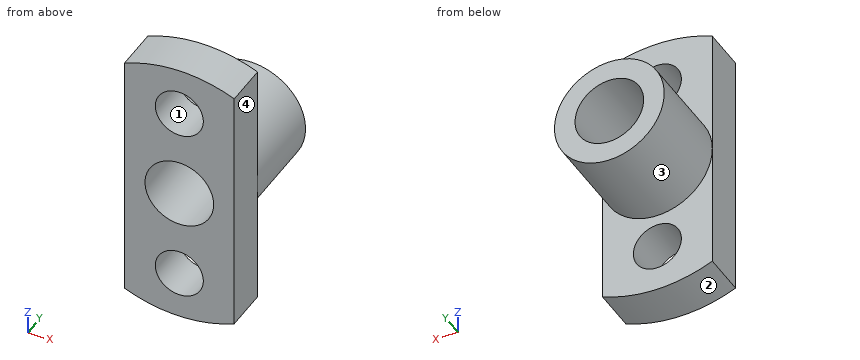
```python
from build123d import *

# Parameters (mm, degrees)
SKETCH_2_R          = 1.75
EXTRUDE_1_DEPTH     = 3.2
SKETCH_3_R          = 4
EXTRUDE_2_DEPTH     = 6.6
SKETCH_4_R          = 2.5
CUT_EXTRUDE_1_DEPTH = 10.8


with BuildPart() as part:
    # 草图2 → 凸台-拉伸1 (new body)
    with BuildSketch(Plane(origin=(0, 0, 0), x_dir=(1, 0, 0), z_dir=(0, 1, 0))):
        with BuildLine():
            Line((-4, 9.16515139), (-4, -9.16515139))
            ThreePointArc((-4, -9.16515139), (0, -10), (4, -9.16515139))
            Line((4, -9.16515139), (4, 9.16515139))
            ThreePointArc((4, 9.16515139), (0, 10), (-4, 9.16515139))
        make_face()
        with Locations((0, 6.5)):
            Circle(SKETCH_2_R, mode=Mode.SUBTRACT)
        with Locations((0, -6.5)):
            Circle(SKETCH_2_R, mode=Mode.SUBTRACT)
    extrude(amount=EXTRUDE_1_DEPTH)

    # 草图3 → 凸台-拉伸2 (add)
    with BuildSketch(Plane(origin=(0, 3.2, 0), x_dir=(1, 0, 0), z_dir=(0, 1, 0))):
        Circle(SKETCH_3_R)
    extrude(amount=EXTRUDE_2_DEPTH)

    # 草图4 → 切除-拉伸1 (cut, through all)
    with BuildSketch(Plane(origin=(0, 9.8, 0), x_dir=(1, 0, 0), z_dir=(0, 1, 0))):
        Circle(SKETCH_4_R)
    extrude(amount=-CUT_EXTRUDE_1_DEPTH, mode=Mode.SUBTRACT)


solid = part.part
```
Could you check a few things on this model? Use its own coordinates, in mm. Face numbers are marked on the shaded views. Round coordinates to 2 decimals unless told otherwise and drop trailing zeros. Order: outer loops, then holes, each group sorted by start corner. A loop starts at its lowest first (then second) coordinate and runs counter-clockwise, first axis right, second up. Notation, with made-up numbers: M 28,89.5 L 39,89.5 A21 cw 39,101.5 Z; hole C 26,-33 d4. An arc over 180 degrees is marked long. One line per question, with ' | ' between items. Start each with the question number.
(1) Suppose I cut it at B-B on x = 0. List the corners of the cut face in (y, z) for me.
(2) Suppose I cut it at D-D on x = -1.25. List the corners of the cut face in (y, z) for me, then the cut area to 3 significant figures.
(3) Suppose I cut it at A-A on z = 6.5. List the corners of the cut face in (x, y) for me.
(4) Suppose I cut it at C-C on y = 6. List the corners of the cut face in (x, z) for me.
(5) Please list where these lines run through material, in increasing order: line 1 along X through (y, z) = (1.85, 6.5); line 2 along Z through (x, y) = (0, 4); line 3 along Z through (x, y) = (-1.25, 1.75).
(6) For P1, Ø4, axis at x = -2, y = 8, coming from the -Z side; P2, Ø2, axis at x = -3, y = 8.5, coming from the -Z side, each with a flat end and sliding along its axis, tell me the tip position at first contact or that it passes through.
(7) Thinking about a two-plate mould opening in Z: for the marked faces 1, 2, 3 and 4, which applies, +Z half, -Z half, draft (parallel to the pull), parting line (faces both ways), or undercut?
Geometry results:
1) outline: M 0,-10 L 3.2,-10 L 3.2,-8.25 L 0,-8.25 Z; M 0,-4.75 L 3.2,-4.75 L 3.2,-4 L 9.8,-4 L 9.8,-2.5 L 0,-2.5 Z; M 0,2.5 L 9.8,2.5 L 9.8,4 L 3.2,4 L 3.2,4.75 L 0,4.75 Z; M 0,8.25 L 3.2,8.25 L 3.2,10 L 0,10 Z
2) outline: M 0,-9.92 L 3.2,-9.92 L 3.2,-7.72 L 0,-7.72 Z; M 0,-5.28 L 3.2,-5.28 L 3.2,-3.8 L 9.8,-3.8 L 9.8,-2.17 L 0,-2.17 Z; M 0,2.17 L 9.8,2.17 L 9.8,3.8 L 3.2,3.8 L 3.2,5.28 L 0,5.28 Z; M 0,7.72 L 3.2,7.72 L 3.2,9.92 L 0,9.92 Z | area: 55.5 mm²
3) outline: M -4,0 L -1.75,0 L -1.75,3.2 L -4,3.2 Z; M 1.75,0 L 4,0 L 4,3.2 L 1.75,3.2 Z
4) outline: C 0,0 d8; hole C 0,0 d5
5) line 1: -4 to -1.75, 1.75 to 4 | line 2: -4 to -2.5, 2.5 to 4 | line 3: -9.92 to -7.72, -5.28 to -2.17, 2.17 to 5.28, 7.72 to 9.92
6) P1: z = -4 | P2: z = -3.46
7) face 1: undercut | face 2: -Z half | face 3: parting line | face 4: draft
